Source: CAD feature listing. Evaluate the final solid. Frame: model axes, mm. A direction names the side the tool comes from. Give positions to 0.01 mm unless a question says otherwise; leave off trailing zeros. Loops run counter-clockwise (first coordinate to the right, second up) from the corner with the lowest first, then second, coordinate; pieces in that order, holes last.
Autodesk Inventor part; units mm, degrees
ref_plane "YZ Plane" through (0, 0, 0) normal (1, 0, 0) x (0, 1, 0)
ref_plane "XZ Plane" through (0, 0, 0) normal (0, 1, 0) x (-1, 0, 0)
ref_plane "XY Plane" through (0, 0, 0) normal (0, 0, 1) x (1, 0, 0)
sketch "Sketch1" plane through (0, 0, 0) normal (0, 1, 0) x (-1, 0, 0)
  circle A0 centre (0, 0) radius 1.5
  dimension "d0" = 3
extrude "Extrusion1" add sketch "Sketch1" along normal blind 61
sketch "Sketch2" plane through (0, 61, 0) normal (0, 1, 0) x (1, 0, 0)
  circle A0 centre (0, 0) radius 1.4
  dimension "d3" = 2.8
extrude "Extrusion2" add sketch "Sketch2" along normal blind 1
sketch "Sketch3" plane through (0, 62, 0) normal (0, 1, 0) x (1, 0, 0)
  circle A0 centre (0, 0) radius 1.5
  dimension "d6" = 3
extrude "Extrusion3" add sketch "Sketch3" along normal blind 10
thread "Thread1"
chamfer "Chamfer1" distance 0.3 angle 45 1 edges at (-1.5, 72, 0)
chamfer "Chamfer2" distance 0.3 angle 45 1 edges at (1.5, 0, 0)
sketch "Sketch4" plane through (0, 0, 0) normal (1, 0, 0) x (0, 1, 0)
  line L0 (62, -1.5) -> (62, 1.5)
  line L1 (71.7, -1.5) -> (71.7, 1.5)
  line L2 (71.7, -1.5) -> (71.7, 1.5)
  line L3 (72, 1.2) -> (72, -1.2)
  line L4 (73.5, 0.5) -> (70.5, 0.5)
  line L5 (70.5, 0.5) -> (70.5, -0.5)
  line L6 (70.5, -0.5) -> (73.5, -0.5)
  line L7 (73.5, -0.5) -> (73.5, 0.5)
  line L8 (72, 1.2) -> (72, -1.2)
  line L9 (73.5, 0.5) -> (70.5, -0.5) construction
  line L10 (70.5, 0.5) -> (73.5, -0.5) construction
  point P0 (0, 0)
  point P1 (72, 0)
  dimension "d17" = 3
  dimension "d18" = 1
extrude "Extrusion4" cut sketch "Sketch4" along normal mid plane 10
properties part number "wał_prowadzący_hamulca" material "Aluminum 6061"
(1) Mould query, pull axis Y, two halves, no side actions, for faces 1 (the flat face through (0, 0, 0)), 2 (the cylindrical face through (-0.325, 66.782, -1.464)), 3 (the cylindrical face through (-1.4, 61.49, 0.06)). Classes: pulls with the +Y half, pulls with the -Y half, needs draft (parallel to the pull), parting line crosses it, or undercut.
A:
face 1: pulls with the -Y half
face 2: needs draft
face 3: undercut
(2) Section A-A, the plane z = 0. Return the cut outline in (x, y).
A:
outline: (-1.5, 0.3) - (-1.2, 0) - (1.2, 0) - (1.5, 0.3) - (1.5, 61) - (1.4, 61) - (1.4, 62) - (1.5, 62) - (1.5, 70.5) - (-1.5, 70.5) - (-1.5, 62) - (-1.4, 62) - (-1.4, 61) - (-1.5, 61) - close
(3) Reachability of faces 4 (the flat face through (0, 71, 0.5)), 5 (the cylindrical face through (1.5, 30.23, -0.07)) from +Z, -Z, +X, -X, +Y, -Y: full face, straight path, thin tool, end or side. Return the list, or none.
A:
face 4: +X, -X, +Y
face 5: +Y, -Y
(4) Ray query, line 1 along Y through (x, z) = (0.65, -0.3); line 2 along X through (y, z) = (51.5, 0.55); line 3 along Z through (x, y) = (-0.9, 20.5). Return the intervals inside material, ascending.
A:
line 1: y = 0 to 70.5
line 2: x = -1.4 to 1.4
line 3: z = -1.2 to 1.2
(5) First-contact query: pin 1 (0.5 mm diameter, centred on x = 0.5, y = 71.5, fed in from -Z). Flat tip, straight axial feed; report the tip coordinate or a pass-through.
A:
pin 1: stops at z = -1.48
(6) Section B-B, the plane y = 13.5. Return the cut outline in (x, z).
A:
outline: circle Ø3 at (0, 0)
